The listing builds one solid part. Answer for the finished solid, in the listing's coordinates (mm). A direction names the side the tool comes from. Coordinates: 2 decimals unless noted, no trailing zeros. Write each loop counter-clockwise with the first axis right and the second up, starting at its lowest first coordinate (ties: lowest second). Pieces come first, ordered by that corner, then holes.
from build123d import *

# Parameters (mm, degrees)
SKETCH1_W           = 50
SKETCH1_H           = 40
BOSS_EXTRUDE1_DEPTH = 27
SKETCH2_W           = 39
SKETCH2_H           = 35
CUT_EXTRUDE1_DEPTH  = 21
SKETCH3_R           = 9
SKETCH3_R_2         = 3.5
SKETCH3_W           = 20
SKETCH3_H           = 3
CUT_EXTRUDE2_DEPTH  = 68.386942355
SKETCH4_R           = 1
CUT_EXTRUDE3_DEPTH  = 6
FILLET1_R           = 1.5


with BuildPart() as part:
    # Sketch1 → Boss-Extrude1 (new body)
    with BuildSketch(Plane.XY):
        with Locations((25, 20)):
            Rectangle(SKETCH1_W, SKETCH1_H)
    extrude(amount=BOSS_EXTRUDE1_DEPTH)

    # Sketch2 → Cut-Extrude1 (cut)
    with BuildSketch(Plane(origin=(0, 0, 0), x_dir=(-1, 0, 0), z_dir=(0, 0, -1))):
        with Locations((-25, 17.5)):
            Rectangle(SKETCH2_W, SKETCH2_H)
    extrude(amount=-CUT_EXTRUDE1_DEPTH, mode=Mode.SUBTRACT)

    # Sketch3 → Cut-Extrude2 (cut, through all)
    with BuildSketch(Plane(origin=(0, 0, 21), x_dir=(-1, 0, 0), z_dir=(0, 0, -1))):
        with Locations((-25, 13.5)):
            Circle(SKETCH3_R)
        with Locations((-39, 25)):
            Circle(SKETCH3_R_2)
        with Locations(Location((-11, 25, 0), (0, 0, 180))):
            Circle(SKETCH3_R_2)
        with Locations((-25, 1.5)):
            Rectangle(SKETCH3_W, SKETCH3_H)
    extrude(amount=-CUT_EXTRUDE2_DEPTH, mode=Mode.SUBTRACT)

    # Sketch4 → Cut-Extrude3 (cut)
    with BuildSketch(Plane.XY.offset(27)):
        with Locations((44.5, 15)):
            Circle(SKETCH4_R)
        with Locations(Location((5.5, 15, 0), (0, 0, 90))):
            Circle(SKETCH4_R)
    extrude(amount=-CUT_EXTRUDE3_DEPTH, mode=Mode.SUBTRACT)

    # Fillet1
    # the kernel refuses this fillet: 1.5 mm, written as the material it adds along each edge
    with BuildSketch(Plane(origin=(15, 3, 21), x_dir=(0, -1, 0), z_dir=(0, 0, 1)), Plane(origin=(35, 3, 21), x_dir=(-1, 0, 0), z_dir=(0, 0, 1))) as fillet1_piece_1:
        with BuildLine():
            CenterArc((FILLET1_R, FILLET1_R), FILLET1_R, 180, 90)
            Line((0, FILLET1_R), (0, 0))
            Line((0, 0), (FILLET1_R, 0))
        make_face()
    extrude(amount=6)
    # the kernel refuses this fillet: 1.5 mm, written as the material it takes off along each edge
    with BuildSketch(Plane(origin=(48.5, 38.5, 1.5), x_dir=(0, 0, -1), z_dir=(1, 0, 0))) as fillet1_2_piece_1_section:
        Polygon((0, 0), (FILLET1_R, 0), (FILLET1_R, FILLET1_R), (0, FILLET1_R), align=None)
    fillet1_2_piece_1 = extrude(amount=FILLET1_R, mode=Mode.PRIVATE)
    fillet1_2_piece_1 = fillet1_2_piece_1 - Plane(origin=(48.5, 38.5, 1.5), x_dir=(0, -0.7071067811865475, 0.7071067811865475), z_dir=(1, 0, 0)) * Sphere(FILLET1_R, mode=Mode.PRIVATE)
    add(fillet1_2_piece_1, mode=Mode.SUBTRACT)
    with BuildSketch(Plane(origin=(1.5, 38.5, 1.5), x_dir=(-1, 0, 0), z_dir=(0, 0, -1))) as fillet1_2_piece_2_section:
        Polygon((0, 0), (FILLET1_R, 0), (FILLET1_R, FILLET1_R), (0, FILLET1_R), align=None)
    fillet1_2_piece_2 = extrude(amount=FILLET1_R, mode=Mode.PRIVATE)
    fillet1_2_piece_2 = fillet1_2_piece_2 - Plane(origin=(1.5, 38.5, 1.5), x_dir=(0.7071067811865475, -0.7071067811865475, 0), z_dir=(0, 0, -1)) * Sphere(FILLET1_R, mode=Mode.PRIVATE)
    add(fillet1_2_piece_2, mode=Mode.SUBTRACT)
    with BuildSketch(Plane(origin=(1.5, 38.5, 25.5), x_dir=(-1, 0, 0), z_dir=(0, 0, 1))) as fillet1_2_piece_3_section:
        Polygon((0, 0), (FILLET1_R, 0), (FILLET1_R, -FILLET1_R), (0, -FILLET1_R), align=None)
    fillet1_2_piece_3 = extrude(amount=FILLET1_R, mode=Mode.PRIVATE)
    fillet1_2_piece_3 = fillet1_2_piece_3 - Plane(origin=(1.5, 38.5, 25.5), x_dir=(0.7071067811865475, -0.7071067811865475, 0), z_dir=(0, 0, 1)) * Sphere(FILLET1_R, mode=Mode.PRIVATE)
    add(fillet1_2_piece_3, mode=Mode.SUBTRACT)
    with BuildSketch(Plane(origin=(48.5, 38.5, 25.5), x_dir=(0, 0, 1), z_dir=(1, 0, 0))) as fillet1_2_piece_4_section:
        Polygon((0, 0), (FILLET1_R, 0), (FILLET1_R, -FILLET1_R), (0, -FILLET1_R), align=None)
    fillet1_2_piece_4 = extrude(amount=FILLET1_R, mode=Mode.PRIVATE)
    fillet1_2_piece_4 = fillet1_2_piece_4 - Plane(origin=(48.5, 38.5, 25.5), x_dir=(0, -0.7071067811865475, -0.7071067811865475), z_dir=(1, 0, 0)) * Sphere(FILLET1_R, mode=Mode.PRIVATE)
    add(fillet1_2_piece_4, mode=Mode.SUBTRACT)
    with BuildSketch(Plane(origin=(15, 0, 17.25), x_dir=(-1, 0, 0), z_dir=(0, 0, 1))) as fillet1_2_piece_5:
        with BuildLine():
            CenterArc((FILLET1_R, -FILLET1_R), FILLET1_R, 90, 90)
            Line((0, -FILLET1_R), (0, 0))
            Line((0, 0), (FILLET1_R, 0))
        make_face()
    extrude(amount=13.5, mode=Mode.SUBTRACT)
    with BuildSketch(Plane(origin=(35, 0, 17.25), x_dir=(1, 0, 0), z_dir=(0, 0, 1))) as fillet1_2_piece_6:
        with BuildLine():
            CenterArc((FILLET1_R, FILLET1_R), FILLET1_R, 180, 90)
            Line((0, FILLET1_R), (0, 0))
            Line((0, 0), (FILLET1_R, 0))
        make_face()
    extrude(amount=13.5, mode=Mode.SUBTRACT)
    with BuildSketch(Plane(origin=(15, -3.75, 21), x_dir=(-1, 0, 0), z_dir=(0, 1, 0)), Plane(origin=(35, 1.5, 21), x_dir=(1, 0, 0), z_dir=(0, -1, 0))) as fillet1_2_piece_7:
        with BuildLine():
            CenterArc((FILLET1_R, FILLET1_R), FILLET1_R, 180, 90)
            Line((0, FILLET1_R), (0, 0))
            Line((0, 0), (FILLET1_R, 0))
        make_face()
    extrude(amount=5.25, mode=Mode.SUBTRACT)
    with BuildSketch(Plane(origin=(16.5, 3, 21), x_dir=(0, 1, 0), z_dir=(1, 0, 0))) as fillet1_2_piece_8:
        with BuildLine():
            CenterArc((FILLET1_R, FILLET1_R), FILLET1_R, 180, 90)
            Line((0, FILLET1_R), (0, 0))
            Line((0, 0), (FILLET1_R, 0))
        make_face()
    extrude(amount=17, mode=Mode.SUBTRACT)
    with BuildSketch(Plane(origin=(39, 25, 21), x_dir=(-1, 0, 0), z_dir=(0, -1, 0))) as fillet1_2_piece_9:
        with BuildLine():
            CenterArc((3.5 + FILLET1_R, -FILLET1_R), FILLET1_R, 90, 90)
            Line((3.5, -FILLET1_R), (3.5, 0))
            Line((3.5, 0), (3.5 + FILLET1_R, 0))
        make_face()
    revolve(axis=Axis((39, 25, 21), (0, 0, -1)), mode=Mode.SUBTRACT)
    with BuildSketch(Plane(origin=(11, 25, 21), x_dir=(1, 0, 0), z_dir=(0, 1, 0))) as fillet1_2_piece_10:
        with BuildLine():
            CenterArc((3.5 + FILLET1_R, -FILLET1_R), FILLET1_R, 90, 90)
            Line((3.5, -FILLET1_R), (3.5, 0))
            Line((3.5, 0), (3.5 + FILLET1_R, 0))
        make_face()
    revolve(axis=Axis((11, 25, 21), (0, 0, -1)), mode=Mode.SUBTRACT)
    with BuildSketch(Plane(origin=(25, 13.5, 21), x_dir=(-1, 0, 0), z_dir=(0, -1, 0))) as fillet1_2_piece_11:
        with BuildLine():
            CenterArc((9 + FILLET1_R, -FILLET1_R), FILLET1_R, 90, 90)
            Line((9, -FILLET1_R), (9, 0))
            Line((9, 0), (9 + FILLET1_R, 0))
        make_face()
    revolve(axis=Axis((25, 13.5, 21), (0, 0, -1)), mode=Mode.SUBTRACT)
    with BuildSketch(Plane(origin=(5.5, -3.75, 0), x_dir=(-1, 0, 0), z_dir=(0, 1, 0)), Plane(origin=(44.5, 35, 0), x_dir=(1, 0, 0), z_dir=(0, -1, 0))) as fillet1_2_piece_12:
        with BuildLine():
            CenterArc((FILLET1_R, FILLET1_R), FILLET1_R, 180, 90)
            Line((0, FILLET1_R), (0, 0))
            Line((0, 0), (FILLET1_R, 0))
        make_face()
    extrude(amount=38.75, mode=Mode.SUBTRACT)
    with BuildSketch(Plane(origin=(5.5, 35, 0), x_dir=(0, 1, 0), z_dir=(1, 0, 0))) as fillet1_2_piece_13:
        with BuildLine():
            CenterArc((FILLET1_R, FILLET1_R), FILLET1_R, 180, 90)
            Line((0, FILLET1_R), (0, 0))
            Line((0, 0), (FILLET1_R, 0))
        make_face()
    extrude(amount=39, mode=Mode.SUBTRACT)
    with BuildSketch(Plane(origin=(50, -3.75, 0), x_dir=(-1, 0, 0), z_dir=(0, 1, 0)), Plane(origin=(0, 38.5, 0), x_dir=(1, 0, 0), z_dir=(0, -1, 0))) as fillet1_2_piece_14:
        with BuildLine():
            CenterArc((FILLET1_R, FILLET1_R), FILLET1_R, 180, 90)
            Line((0, FILLET1_R), (0, 0))
            Line((0, 0), (FILLET1_R, 0))
        make_face()
    extrude(amount=42.25, mode=Mode.SUBTRACT)
    with BuildSketch(Plane(origin=(48.5, 40, 0), x_dir=(0, -1, 0), z_dir=(-1, 0, 0))) as fillet1_2_piece_15:
        with BuildLine():
            CenterArc((FILLET1_R, FILLET1_R), FILLET1_R, 180, 90)
            Line((0, FILLET1_R), (0, 0))
            Line((0, 0), (FILLET1_R, 0))
        make_face()
    extrude(amount=47, mode=Mode.SUBTRACT)
    with BuildSketch(Plane(origin=(0, 40, 1.5), x_dir=(0, -1, 0), z_dir=(0, 0, 1)), Plane(origin=(50, 40, 1.5), x_dir=(-1, 0, 0), z_dir=(0, 0, 1))) as fillet1_2_piece_16:
        with BuildLine():
            CenterArc((FILLET1_R, FILLET1_R), FILLET1_R, 180, 90)
            Line((0, FILLET1_R), (0, 0))
            Line((0, 0), (FILLET1_R, 0))
        make_face()
    extrude(amount=24, mode=Mode.SUBTRACT)
    with BuildSketch(Plane(origin=(0, 38.5, 27), x_dir=(1, 0, 0), z_dir=(0, -1, 0)), Plane(origin=(50, -3.75, 27), x_dir=(-1, 0, 0), z_dir=(0, 1, 0))) as fillet1_2_piece_17:
        with BuildLine():
            CenterArc((FILLET1_R, -FILLET1_R), FILLET1_R, 90, 90)
            Line((0, -FILLET1_R), (0, 0))
            Line((0, 0), (FILLET1_R, 0))
        make_face()
    extrude(amount=42.25, mode=Mode.SUBTRACT)
    with BuildSketch(Plane(origin=(48.5, 40, 27), x_dir=(0, -1, 0), z_dir=(-1, 0, 0))) as fillet1_2_piece_18:
        with BuildLine():
            CenterArc((FILLET1_R, -FILLET1_R), FILLET1_R, 90, 90)
            Line((0, -FILLET1_R), (0, 0))
            Line((0, 0), (FILLET1_R, 0))
        make_face()
    extrude(amount=47, mode=Mode.SUBTRACT)
    with BuildSketch(Plane(origin=(16.5, 1.5, 21), x_dir=(-1, 0, 0), z_dir=(0, -1, 0))) as fillet1_2_piece_19:
        with BuildLine():
            CenterArc((1.5 + FILLET1_R, -FILLET1_R), FILLET1_R, 90, 90)
            Line((1.5, -FILLET1_R), (1.5, 0))
            Line((1.5, 0), (1.5 + FILLET1_R, 0))
        make_face()
    revolve(axis=Axis((16.5, 1.5, 21), (0, 0, -1)), revolution_arc=90, mode=Mode.SUBTRACT)
    with BuildSketch(Plane(origin=(33.5, 1.5, 21), x_dir=(0, 1, 0), z_dir=(-1, 0, 0))) as fillet1_2_piece_20:
        with BuildLine():
            CenterArc((1.5 + FILLET1_R, -FILLET1_R), FILLET1_R, 90, 90)
            Line((1.5, -FILLET1_R), (1.5, 0))
            Line((1.5, 0), (1.5 + FILLET1_R, 0))
        make_face()
    revolve(axis=Axis((33.5, 1.5, 21), (0, 0, -1)), revolution_arc=90, mode=Mode.SUBTRACT)
    with BuildSketch(Plane(origin=(1.75, 35, 0), x_dir=(0, 1, 0), z_dir=(1, 0, 0))) as fillet1_2_piece_21a_section:
        with BuildLine():
            CenterArc((FILLET1_R, FILLET1_R), FILLET1_R, 180, 90)
            Line((0, FILLET1_R), (0, 0))
            Line((0, 0), (FILLET1_R, 0))
        make_face()
    fillet1_2_piece_21a = extrude(amount=42.75, mode=Mode.PRIVATE)
    fillet1_2_piece_21a = split(fillet1_2_piece_21a, bisect_by=Plane(origin=(5.5, 35.339592671, 0.339592671), z_dir=(-1, 0, 0)), keep=Keep.TOP, mode=Mode.PRIVATE)
    with BuildSketch(Plane(origin=(5.5, -3.75, 0), x_dir=(-1, 0, 0), z_dir=(0, 1, 0))) as fillet1_2_piece_21b_section:
        with BuildLine():
            CenterArc((FILLET1_R, FILLET1_R), FILLET1_R, 180, 90)
            Line((0, FILLET1_R), (0, 0))
            Line((0, 0), (FILLET1_R, 0))
        make_face()
    fillet1_2_piece_21b = extrude(amount=42.5, mode=Mode.PRIVATE)
    fillet1_2_piece_21b = split(fillet1_2_piece_21b, bisect_by=Plane(origin=(5.160407329, 35, 0.339592671), z_dir=(0, 1, 0)), keep=Keep.TOP, mode=Mode.PRIVATE)
    fillet1_2_piece_21 = fillet1_2_piece_21a & fillet1_2_piece_21b
    add(fillet1_2_piece_21, mode=Mode.SUBTRACT)
    with BuildSketch(Plane(origin=(44.5, 38.75, 0), x_dir=(1, 0, 0), z_dir=(0, -1, 0))) as fillet1_2_piece_22a_section:
        with BuildLine():
            CenterArc((FILLET1_R, FILLET1_R), FILLET1_R, 180, 90)
            Line((0, FILLET1_R), (0, 0))
            Line((0, 0), (FILLET1_R, 0))
        make_face()
    fillet1_2_piece_22a = extrude(amount=42.5, mode=Mode.PRIVATE)
    fillet1_2_piece_22a = split(fillet1_2_piece_22a, bisect_by=Plane(origin=(44.839592671, 35, 0.339592671), z_dir=(0, 1, 0)), keep=Keep.TOP, mode=Mode.PRIVATE)
    with BuildSketch(Plane(origin=(5.5, 35, 0), x_dir=(0, 1, 0), z_dir=(1, 0, 0))) as fillet1_2_piece_22b_section:
        with BuildLine():
            CenterArc((FILLET1_R, FILLET1_R), FILLET1_R, 180, 90)
            Line((0, FILLET1_R), (0, 0))
            Line((0, 0), (FILLET1_R, 0))
        make_face()
    fillet1_2_piece_22b = extrude(amount=42.75, mode=Mode.PRIVATE)
    fillet1_2_piece_22b = split(fillet1_2_piece_22b, bisect_by=Plane(origin=(44.5, 35.339592671, 0.339592671), z_dir=(1, 0, 0)), keep=Keep.TOP, mode=Mode.PRIVATE)
    fillet1_2_piece_22 = fillet1_2_piece_22a & fillet1_2_piece_22b
    add(fillet1_2_piece_22, mode=Mode.SUBTRACT)


solid = part.part
1. A tool of negligible diameter and unlimited length cuts with its end or side. For faces 1 (the flat face through (5.5, 17, 11)), 2 (the cylindrical face through (5.2, 15.954, 24.042)), 3 (the flat face through (25, 3, 25)), from which of +Z, -Z, +X, -X, +Y, -Y can it reach the whole face along a straight path? Write none if from no direction.
Results found:
face 1: -Z, -Y
face 2: +Z
face 3: +Z, -Z, -Y
2. Section B-B on z = 7.5 is taken. Give the vertices of the cut face in (x, y).
Results found:
outline: (0, 0) - (5.5, 0) - (5.5, 35) - (44.5, 35) - (44.5, 0) - (50, 0) - (50, 38.5) arc R1.5 ccw to (48.5, 40) - (1.5, 40) arc R1.5 ccw to (0, 38.5) - close
3. Section A-A on x = 39 is taken. Give the vertices of the cut face in (y, z).
Results found:
outline: (0, 21) - (20, 21) arc R1.5 ccw to (21.5, 22.5) - (21.5, 27) - (0, 27) - close; (28.5, 22.5) arc R1.5 ccw to (30, 21) - (35, 21) - (35, 1.5) arc R1.5 ccw to (36.5, 0) - (38.5, 0) arc R1.5 ccw to (40, 1.5) - (40, 25.5) arc R1.5 ccw to (38.5, 27) - (28.5, 27) - close
4. Section C-C on y = 31 is taken. Give the vertices of the cut face in (x, z).
Results found:
outline: (0, 1.5) arc R1.5 ccw to (1.5, 0) - (4, 0) arc R1.5 ccw to (5.5, 1.5) - (5.5, 21) - (44.5, 21) - (44.5, 1.5) arc R1.5 ccw to (46, 0) - (48.5, 0) arc R1.5 ccw to (50, 1.5) - (50, 25.5) arc R1.5 ccw to (48.5, 27) - (1.5, 27) arc R1.5 ccw to (0, 25.5) - close
5. Flat-ended cylindrical pins translate along their axes: P1, Ø1.2, axis at x = 5.5, y = 15, coming from the +Z side; P2, Ø2, axis at x = 27.5, z = 24, coming from the -Y side; P3, Ø1.2, axis at x = 44.5, y = 15, coming from the -Z side; P4, Ø6, axis at y = 8, z = 16.5, coming from the -X side. Find the tip coordinate at first contact, or state that the pin passes through.
Results found:
P1: stops at z = 21
P2: stops at y = 3
P3: stops at z = 0.3
P4: stops at x = 0
6. Find the intervals of material crossed by L1, parallel to X at y = 15, z = 23.85; L2, parallel to X at y = 12.5, z = 14.75; L3, parallel to Y at x = 42.5, z = 15.5, in increasing order.
Results found:
L1: x = 0 to 4.5, 6.5 to 16.13, 33.87 to 43.5, 45.5 to 50
L2: x = 0 to 5.5, 44.5 to 50
L3: y = 35 to 40
7. Section D-D on y = 15 is taken. State how many separate pieces and enclosed holes the cut face has, then the cut area to 3 significant figures.
Results found:
separate pieces: 4
enclosed holes: 0
area: 397 mm2
